```python
from build123d import *

# Parameters (mm, degrees)
SKETCH_1_R          = 2.1
SKETCH_1_R_2        = 1.5
EXTRUDE_1_DEPTH     = 4
SKETCH_1_3_W        = 6
SKETCH_1_3_H        = 12
EXTRUDE_2_DEPTH     = 9
FILLET_1_R          = 2
CUT_EXTRUDE_START   = -5
CUT_EXTRUDE_1_DEPTH = 10


with BuildPart() as part:
    # 草图1 → 凸台-拉伸1 (new body)
    with BuildSketch(Plane.XY):
        Polygon((0, 22), (0, 0), (20, 0), (20, 22), (13, 22), (13, 10), (7, 10), (7, 22), align=None)
        with Locations((10, 4)):
            Circle(SKETCH_1_R, mode=Mode.SUBTRACT)
        with Locations((5, 17)):
            Circle(SKETCH_1_R_2, mode=Mode.SUBTRACT)
        with Locations((15, 17)):
            Circle(SKETCH_1_R_2, mode=Mode.SUBTRACT)
    extrude(amount=EXTRUDE_1_DEPTH)

    # 草图1<3> → 凸台-拉伸2 (add)
    with BuildSketch(Plane.XY):
        with Locations((10, 16)):
            Rectangle(SKETCH_1_3_W, SKETCH_1_3_H)
    extrude(amount=EXTRUDE_2_DEPTH)

    # 圆角1
    fillet_1_edges = [part.edges().sort_by_distance(p)[0] for p in [
        (20, 22, 2),
        (20, 0, 2),
        (0, 0, 2),
        (0, 22, 2),
    ]]
    fillet(fillet_1_edges, radius=FILLET_1_R)

    # 草图2 → 切除-拉伸1 (cut)
    with BuildSketch(Plane.ZY.offset(CUT_EXTRUDE_START)):
        Polygon((2.8, 18.5), (4, 18.5), (14, 18.5), (14, 15.5), (4, 15.5), (2.8, 15.5), align=None)
    extrude(amount=-CUT_EXTRUDE_1_DEPTH, mode=Mode.SUBTRACT)


solid = part.part
```
Design review of the part built by this model. Coordinates are the model's own, in mm. A direction names the side the tool comes from. Give positions to 0.01 mm unless a question says otherwise; leave off trailing zeros. Order: outer loops, then holes, each group sorted by start corner. A loop starts at its lowest first (then second) coordinate and runs counter-clockwise, first axis right, second up. Notation, with made-up numbers: (19.5, 19) -> (51.5, 19) arc R23 ccw to (51.5, 43) -> close; hole circle Ø6 at (8, 52.5). An arc over 180 degrees is marked (long way). Write item = value, one per line. Start each with the question number.
(1) We need section A-A on x = 10. Write out the cut boundary in (y, z), plus the area to 3 significant figures.
(2) We need section D-D on z = 3.5. Write out the cut boundary in (x, y), plus the area to 3 significant figures.
(3) To check wall thickness, follow line 1 along X through (y, z) = (17, 1.6); line 2 along Y through (x, z) = (15, 0.9); line 3 along X through (y, z) = (18.25, 2.5). State the ranges of each line that lie inside material, in increasing order.
(4) We need section C-C on y = 4. Write out the cut boundary in (x, z), plus the area to 3 significant figures.
(5) For faces 1 (the face through (7, 13, 6)), 2 (the face through (13, 20, 6)), 3 (the face through (10, 22, 3)), 4 (the face through (10, 15.5, 5)), list the 3-axis set-ups (+Z, -Z, +X, -X, +Y, -Y) from which the entire face can be reached by the end or side of a thin tool; tool diameter is ignored.
(6) We need section B-B on z = 1. Write out the cut boundary in (x, y).
(7) For pin 1 (2.5 mm diameter, centred on x = 15, y = 17, fed in from -Z); pin 2 (4 mm diameter, centred on y = 19.5, z = 7, fed in from -X); pin 3 (5.5 mm diameter, centred on x = 10, y = 4, fed in from +Z); pin 4 (3 mm diameter, centred on y = 20.5, z = 6, fed in from +X), all flat-tipped, find the tip position at first contact; note any pin that passes through.
(8) Mouldability with a two-part tool opening along X and no side actions: class faces 5 (the face through (10, 0, 2)), 6 (the face through (10, 18.5, 5)), 7 (the face through (13, 13, 6)) as +X half, -X half, draft (parallel to the pull), parting line (faces both ways), or undercut.
Numbers:
q1.outline = (0, 0) -> (1.9, 0) -> (1.9, 4) -> (0, 4) -> close; (6.1, 0) -> (22, 0) -> (22, 9) -> (18.5, 9) -> (18.5, 2.8) -> (15.5, 2.8) -> (15.5, 9) -> (10, 9) -> (10, 4) -> (6.1, 4) -> close
q1.area = 113 mm^2
q2.outline = (0, 2) arc R2 ccw to (2, 0) -> (18, 0) arc R2 ccw to (20, 2) -> (20, 20) arc R2 ccw to (18, 22) -> (2, 22) arc R2 ccw to (0, 20) -> close; hole (5, 15.5) -> (15, 15.5) arc R1.5 ccw to (15, 18.5) -> (5, 18.5) arc R1.5 ccw to start; hole circle Ø4.2 at (10, 4)
q2.area = 386 mm^2
q3.line_1 = 0 to 3.5, 6.5 to 13.5, 16.5 to 20
q3.line_2 = 0 to 15.5, 18.5 to 22
q3.line_3 = 0 to 4.17, 5.83 to 14.17, 15.83 to 20
q4.outline = (0, 0) -> (7.9, 0) -> (7.9, 4) -> (0, 4) -> close; (12.1, 0) -> (20, 0) -> (20, 4) -> (12.1, 4) -> close
q4.area = 63.2 mm^2
q5.face_1 = +Z, -X, +Y, -Y
q5.face_2 = +Z, +X, +Y, -Y
q5.face_3 = +Z, -Z, +X, -X, +Y
q5.face_4 = +Z
q6.outline = (0, 2) arc R2 ccw to (2, 0) -> (18, 0) arc R2 ccw to (20, 2) -> (20, 20) arc R2 ccw to (18, 22) -> (2, 22) arc R2 ccw to (0, 20) -> close; hole circle Ø3 at (5, 17); hole circle Ø4.2 at (10, 4); hole circle Ø3 at (15, 17)
q7.pin_1 = through
q7.pin_2 = 7
q7.pin_3 = 4
q7.pin_4 = 13
q8.face_5 = draft
q8.face_6 = undercut
q8.face_7 = +X half
